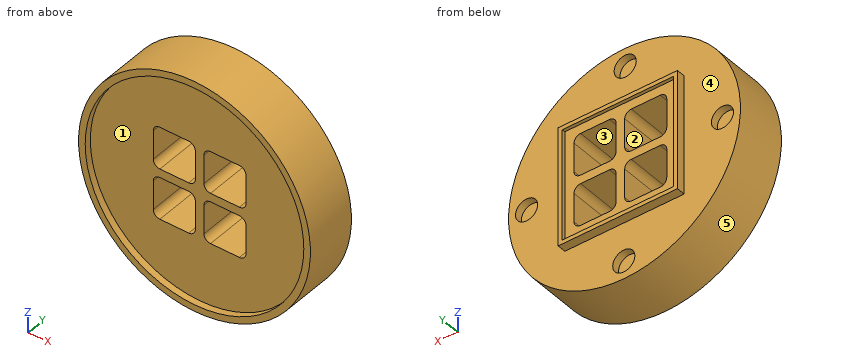
```python
from build123d import *

# Parameters (mm, degrees)
SKETCH1_R           = 17.5
BOSS_EXTRUDE1_DEPTH = 8
SKETCH5_R           = 16.5
CUT_EXTRUDE2_DEPTH  = 1
SKETCH11_R          = 1.67
CUT_EXTRUDE5_DEPTH  = 1.15
CIRPATTERN1_COUNT   = 4
SKETCH13_W          = 18
SKETCH13_H          = 18
SKETCH13_W_2        = 16.8
SKETCH13_H_2        = 16.8
BOSS_EXTRUDE3_DEPTH = 1.3
SKETCH12_W          = 18
SKETCH12_H          = 18
SKETCH12_W_2        = 14
SKETCH12_H_2        = 14
SKETCH12_W_3        = 6.349092008
SKETCH12_H_3        = 1.301815984
SKETCH12_W_4        = 1.301815984
SKETCH12_H_4        = 6.349092008
BOSS_EXTRUDE2_DEPTH = 0.8
SKETCH14_W          = 6.349092008
SKETCH14_H          = 6.349092008
CUT_EXTRUDE6_DEPTH  = 27.009613607
FILLET1_R           = 1


with BuildPart() as part:
    # Sketch1 → Boss-Extrude1 (new body)
    with BuildSketch(Plane(origin=(0, 0, 0), x_dir=(1, 0, 0), z_dir=(0, 1, 0))):
        with Locations(Location((0, 0, 0), (0, 0, 270))):
            Circle(SKETCH1_R)
    extrude(amount=BOSS_EXTRUDE1_DEPTH)

    # Sketch5 → Cut-Extrude2 (cut)
    with BuildSketch(Plane.XZ):
        with Locations(Location((0, 0, 0), (0, 0, 270))):
            Circle(SKETCH5_R)
    extrude(amount=-CUT_EXTRUDE2_DEPTH, mode=Mode.SUBTRACT)

    # Sketch11 → Cut-Extrude5 (cut)
    with BuildSketch(Plane(origin=(0, 8, 0), x_dir=(1, 0, 0), z_dir=(0, 1, 0))):
        with Locations(Location((0.106708516, 14.783412681, 0), (0, 0, 270))):
            Circle(SKETCH11_R)
    cut_extrude5 = extrude(amount=-CUT_EXTRUDE5_DEPTH, mode=Mode.SUBTRACT)

    # CirPattern1: Cut-Extrude5 ×4 about axis
    cirpattern1_axis = Axis((0, 0, 0), (0, 1, 0))
    for i in range(1, CIRPATTERN1_COUNT):
        add(cut_extrude5.rotate(cirpattern1_axis, i * 360 / CIRPATTERN1_COUNT), mode=Mode.SUBTRACT)

    # Sketch13 → Boss-Extrude3 (add)
    with BuildSketch(Plane(origin=(0, 8, 0), x_dir=(1, 0, 0), z_dir=(0, 1, 0))):
        Rectangle(SKETCH13_W, SKETCH13_H)
        Rectangle(SKETCH13_W_2, SKETCH13_H_2, mode=Mode.SUBTRACT)
    extrude(amount=BOSS_EXTRUDE3_DEPTH)

    # Sketch12 → Boss-Extrude2 (add)
    # profile 1 of 6: a face of its own
    with BuildSketch(Plane(origin=(0, 8, 0), x_dir=(1, 0, 0), z_dir=(0, 1, 0))):
        Rectangle(SKETCH12_W, SKETCH12_H)
        Rectangle(SKETCH12_W_2, SKETCH12_H_2, mode=Mode.SUBTRACT)
    # profile 2 of 6: a face of its own
    with BuildSketch(Plane(origin=(0, 8, 0), x_dir=(1, 0, 0), z_dir=(0, 1, 0))):
        with Locations((-3.825453996, 0)):
            Rectangle(SKETCH12_W_3, SKETCH12_H_3)
    # profile 3 of 6: a face of its own
    with BuildSketch(Plane(origin=(0, 8, 0), x_dir=(1, 0, 0), z_dir=(0, 1, 0))):
        with Locations((0, 3.825453996)):
            Rectangle(SKETCH12_W_4, SKETCH12_H_4)
    # profile 4 of 6: a face of its own
    with BuildSketch(Plane(origin=(0, 8, 0), x_dir=(1, 0, 0), z_dir=(0, 1, 0))):
        with Locations((0, -3.825453996)):
            Rectangle(SKETCH12_W_4, SKETCH12_H_4)
    # profile 5 of 6: a face of its own
    with BuildSketch(Plane(origin=(0, 8, 0), x_dir=(1, 0, 0), z_dir=(0, 1, 0))):
        Rectangle(SKETCH12_W_4, SKETCH12_H_3)
    # profile 6 of 6: a face of its own
    with BuildSketch(Plane(origin=(0, 8, 0), x_dir=(1, 0, 0), z_dir=(0, 1, 0))):
        with Locations((3.825453996, 0)):
            Rectangle(SKETCH12_W_3, SKETCH12_H_3)
    extrude(amount=BOSS_EXTRUDE2_DEPTH)

    # Sketch14 → Cut-Extrude6 (cut, through all)
    with BuildSketch(Plane(origin=(0, 8, 0), x_dir=(1, 0, 0), z_dir=(0, 1, 0))):
        with Locations((-3.825453996, 3.825453996)):
            Rectangle(SKETCH14_W, SKETCH14_H)
        with Locations((-3.825453996, -3.825453996)):
            Rectangle(SKETCH14_W, SKETCH14_H)
        with Locations((3.825453996, -3.825453996)):
            Rectangle(SKETCH14_W, SKETCH14_H)
        with Locations((3.825453996, 3.825453996)):
            Rectangle(SKETCH14_W, SKETCH14_H)
    extrude(amount=-CUT_EXTRUDE6_DEPTH, mode=Mode.SUBTRACT)

    # Fillet1
    fillet1_edges = [part.edges().sort_by_distance(p)[0] for p in [
        (-7, 4.9, 0.650907992),
        (-0.650907992, 4.9, 0.650907992),
        (-0.650907992, 4.9, 7),
        (-0.650907992, 4.5, -7),
        (-0.650907992, 4.5, -0.650907992),
        (-7, 4.9, -0.650907992),
        (0.650907992, 4.9, 7),
        (0.650907992, 4.9, 0.650907992),
        (7, 4.5, 0.650907992),
        (7, 4.9, -0.650907992),
        (0.650907992, 4.9, -0.650907992),
        (0.650907992, 4.9, -7),
        (-7, 4.9, -7),
        (7, 4.5, 7),
        (7, 4.9, -7),
        (-7, 4.9, 7),
    ]]
    fillet(fillet1_edges, radius=FILLET1_R)


solid = part.part
```
The listing builds one solid part. Answer for the finished solid, in the listing's coordinates (mm). Face numbers are marked on the shaded views. A direction names the side the tool comes from. Coordinates: 2 decimals unless noted, no trailing zeros. Write each loop counter-clockwise with the first axis right and the second up, starting at its lowest first coordinate (ties: lowest second). Pieces come first, ordered by that corner, then holes. Notation, with made-up numbers: (-9.75, 35.25) -> (16.25, 35.25) arc R26 cw to (16.25, 66.25) -> close; hole circle Ø9 at (-27, 5.5). An arc over 180 degrees is marked (long way). Write each question's results on one line, items separated by ' | '. Start each with the question number.
1) A cutting plane is placed at C-C (x = 11). Determine the outline of the cut face in (y, z).
2) A tool of negligible diameter and unlimited length cuts with its end or side. For the marked faces 1 and 2, from which of +Z, -Z, +X, -X, +Y, -Y can it reach the whole face along a straight path? Write none if from no direction.
3) Straight lines are drawn through the part: probe 1 along X at (y, z) = (8.25, -4); probe 2 along X at (y, z) = (0.85, 0); probe 3 along Z at (x, y) = (-3, 1.25). For each, find the intervals that lie inside material, in ascending order.
4) A cutting plane is placed at A-A (y = 6). Count the separate pieces of the cut face and the enclosed holes in it, then the cut area to 3 significant figures.
5) Flat-ended cylindrical pins translate along their axes: pin 1 Ø5 at (x, y) = (4.5, 5.5) entering from -Z; pin 2 Ø5 at (y, z) = (6, 12.5) entering from +X; pin 3 Ø1.4 at (y, z) = (8.5, 1) entering from -X. Find the tip coordinate at first contact, or state that the pin passes through.
6) For a pull along Z with two mould halves and no side action, classify the marked faces 3, 4 and 5 as +Z half, -Z half, draft (parallel to the pull), parting line (faces both ways), or undercut.
7) A cutting plane is placed at B-B (z = -3). Determine the outline of the cut face in (x, y), then the cut area to 3 significant figures.
8) A cutting plane is placed at D-D (z = -14.5). Determine the outline of the cut face in (x, y), then the cut area to 3 significant figures.
Values follow:
1) outline: (0, -13.61) -> (8, -13.61) -> (8, 13.61) -> (0, 13.61) -> (0, 12.3) -> (1, 12.3) -> (1, -12.3) -> (0, -12.3) -> close
2) face 1: -Y | face 2: +Y, -Y
3) probe 1: -9 to -7, -0.65 to 0.65, 7 to 9 | probe 2: -17.5 to -16.5, 16.5 to 17.5 | probe 3: -17.24 to -7, -0.65 to 0.65, 7 to 17.24
4) separate pieces: 1 | enclosed holes: 4 | area: 804 mm²
5) pin 1: z = -17.39 | pin 2: x = 14.36 | pin 3: x = -17.49
6) face 3: undercut | face 4: draft | face 5: parting line
7) outline: (-17.24, 0) -> (-16.22, 0) -> (-16.22, 1) -> (-7, 1) -> (-7, 8.8) -> (-8.4, 8.8) -> (-8.4, 9.3) -> (-9, 9.3) -> (-9, 8) -> (-17.24, 8) -> close; (-0.65, 1) -> (0.65, 1) -> (0.65, 8.8) -> (-0.65, 8.8) -> close; (7, 1) -> (16.22, 1) -> (16.22, 0) -> (17.24, 0) -> (17.24, 8) -> (9, 8) -> (9, 9.3) -> (8.4, 9.3) -> (8.4, 8.8) -> (7, 8.8) -> close | area: 159 mm²
8) outline: (-9.8, 0) -> (-7.87, 0) -> (-7.87, 1) -> (7.87, 1) -> (7.87, 0) -> (9.8, 0) -> (9.8, 8) -> (1.75, 8) -> (1.75, 6.85) -> (-1.54, 6.85) -> (-1.54, 8) -> (-9.8, 8) -> close | area: 137 mm²
